Drawing for the job (mm, zero at the part's lowest x, y, z). Coordinates: 2 decimals unless noted, no trailing zeros. Order: outer loops, then holes, each group sorted by start corner. A loop starts at its lowest first (then second) coordinate and runs counter-clockwise, first axis right, second up.
1) Wall check: L1, parallel to X at y = 10, z = 5 (1 decimal); L2, parallel to X at y = 10.75, z = 15.75 (1 decimal); L3, parallel to X at y = 6.5, z = 4.25. Give the ranges that are in metal, low to high.
2) Mould opens along Y. For the marked faces 1, 2, 3 and 4 say: +Y half, -Y half, draft (parallel to the pull), parting line (faces both ways), or undercut.
3) Pin check, flat tips, straight feed: pin 1 Ø1.5 at (x, z) = (8, 2.5) entering from -Y; pin 2 Ø4 at (x, z) = (1.5, 6.5) entering from +Y (1 decimal); pin 3 Ø1.3 at (y, z) = (10.5, 6) entering from +X. Stop position of each tip, or through.
4) Cut at D-D (y = 12). List the corners of the cut face in (x, z).
5) Cut at B-B (x = 3). List the corners of the cut face in (y, z).
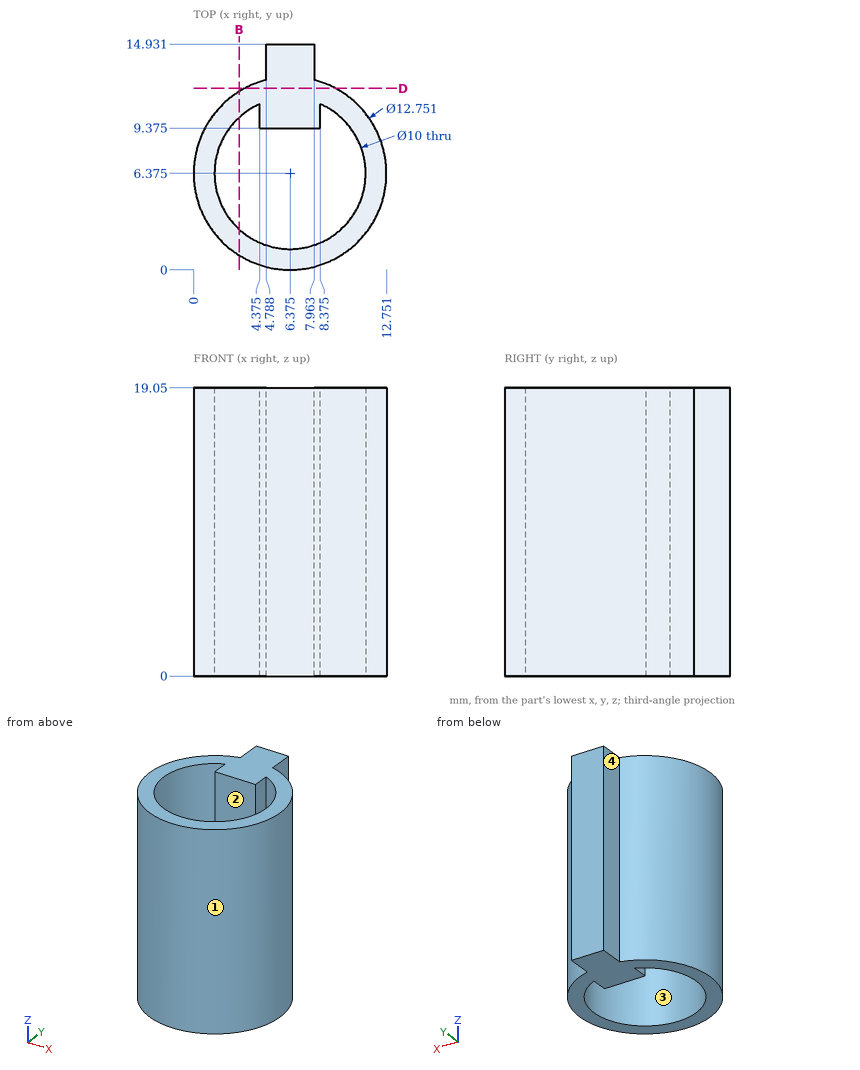
Geometry check:
1. L1: x = 1.1 to 2.9, 4.4 to 8.4, 9.8 to 11.6
1. L2: x = 1.7 to 4, 4.4 to 8.4, 8.8 to 11
1. L3: x = 0 to 1.38, 11.37 to 12.75
2. face 1: parting line
2. face 2: undercut
2. face 3: undercut
2. face 4: draft
3. pin 1: stops at y = 0.06
3. pin 2: stops at y = 12.1
3. pin 3: stops at x = 11.72
4. outline: (3.37, 0) - (9.38, 0) - (9.38, 19.05) - (3.37, 19.05) - close
5. outline: (0.97, 0) - (2.69, 0) - (2.69, 19.05) - (0.97, 19.05) - close; (10.06, 0) - (11.78, 0) - (11.78, 19.05) - (10.06, 19.05) - close
